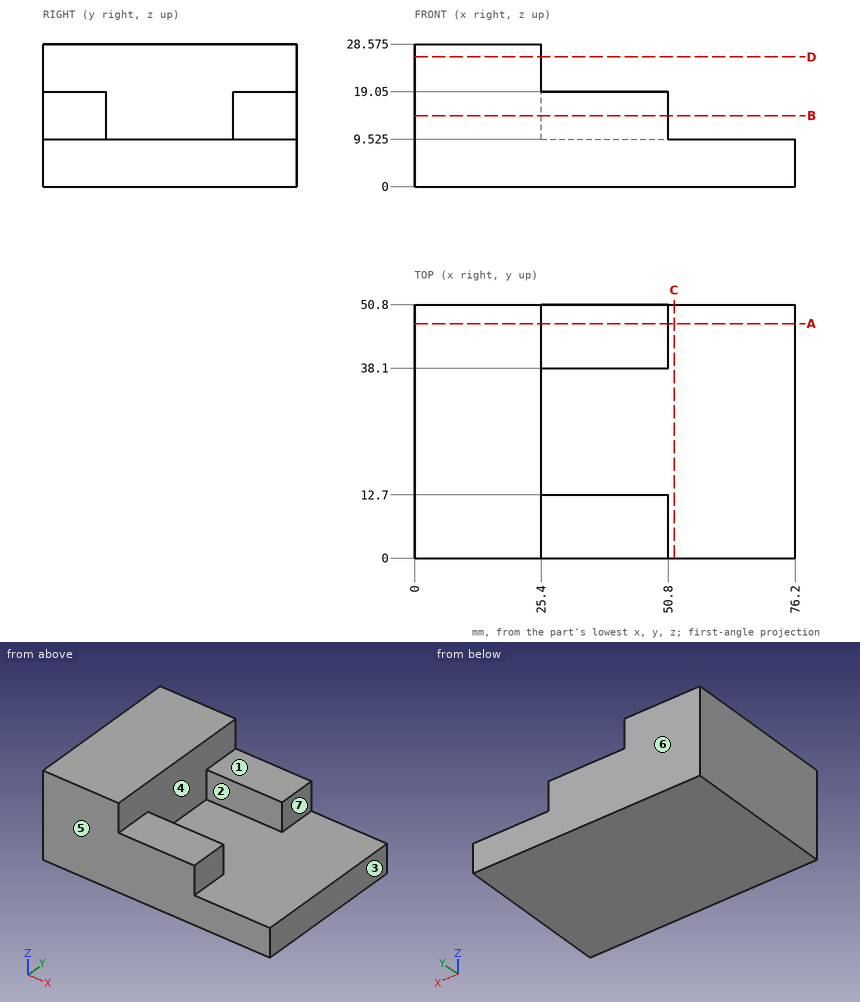
The figure shows three views and two pictorial views of one solid part (mm, origin at its lowest corner). Answer the questions. A direction names the side the tool comes from. Coordinates: 2 decimals unless noted, no trailing zeros. Loops run counter-clockwise (first coordinate to the right, second up) from the corner with the lowest first, then second, coordinate; pieces in that order, holes last.
1) Find section D-D on z = 26. Write down the section's boundary in (x, y).
2) Determine the mould class of the marked faces 4, 5, 6 and 7 for opening direction Y: pulls with the +Y half, pulls with the -Y half, needs draft (parallel to the pull), parting line crosses it, or undercut.
3) Find section C-C on x = 52. Write down the section's boundary in (y, z) (3 decimals), then the cut area to 3 significant figures.
4) A tool of negligible diameter and unlimited length cuts with its end or side. For the marked faces 1, 2 and 3, from which of +Z, -Z, +X, -X, +Y, -Y can it reach the whole face along a straight path? Write none if from no direction.
5) Find section B-B on z = 14.25. Write down the section's boundary in (x, y), then the cut area to 3 significant figures.
6) Find the intervals of material crossed by L1, parallel to Y at x = 29, z = 10.25; L2, parallel to X at y = 43, z = 18.5; L3, parallel to X at y = 33, z = 16.5, in increasing order.
7) Find section A-A on y = 47. Write down the section's boundary in (x, z) (3 decimals), then the cut area to 3 significant figures.
8) Flat-ended cylindrical pins translate along their axes: pin 1 Ø3 at (y, z) = (45.5, 14.5) entering from +X; pin 2 Ø10 at (x, z) = (56, 23.5) entering from -Y; pin 3 Ø5 at (x, y) = (25, 10.5) entering from -Z; pin 4 Ø15 at (x, y) = (60.5, 13) entering from +Z (3 decimals). Find the tip coordinate at first contact, or state that the pin passes through.
Values:
1. outline: (0, 0) - (25.4, 0) - (25.4, 50.8) - (0, 50.8) - close
2. face 4: undercut
2. face 5: pulls with the -Y half
2. face 6: pulls with the +Y half
2. face 7: needs draft
3. outline: (0, 0) - (50.8, 0) - (50.8, 9.525) - (0, 9.525) - close
3. area: 484 mm2
4. face 1: +Z, +X, +Y, -Y
4. face 2: +Z, +X
4. face 3: +Z, -Z, +X, +Y, -Y
5. outline: (0, 0) - (50.8, 0) - (50.8, 12.7) - (25.4, 12.7) - (25.4, 38.1) - (50.8, 38.1) - (50.8, 50.8) - (0, 50.8) - close
5. area: 1,940 mm2
6. L1: y = 0 to 12.7, 38.1 to 50.8
6. L2: x = 0 to 50.8
6. L3: x = 0 to 25.4
7. outline: (0, 0) - (76.2, 0) - (76.2, 9.525) - (50.8, 9.525) - (50.8, 19.05) - (25.4, 19.05) - (25.4, 28.575) - (0, 28.575) - close
7. area: 1,450 mm2
8. pin 1: stops at x = 50.8
8. pin 2: passes through
8. pin 3: stops at z = 0
8. pin 4: stops at z = 9.525
